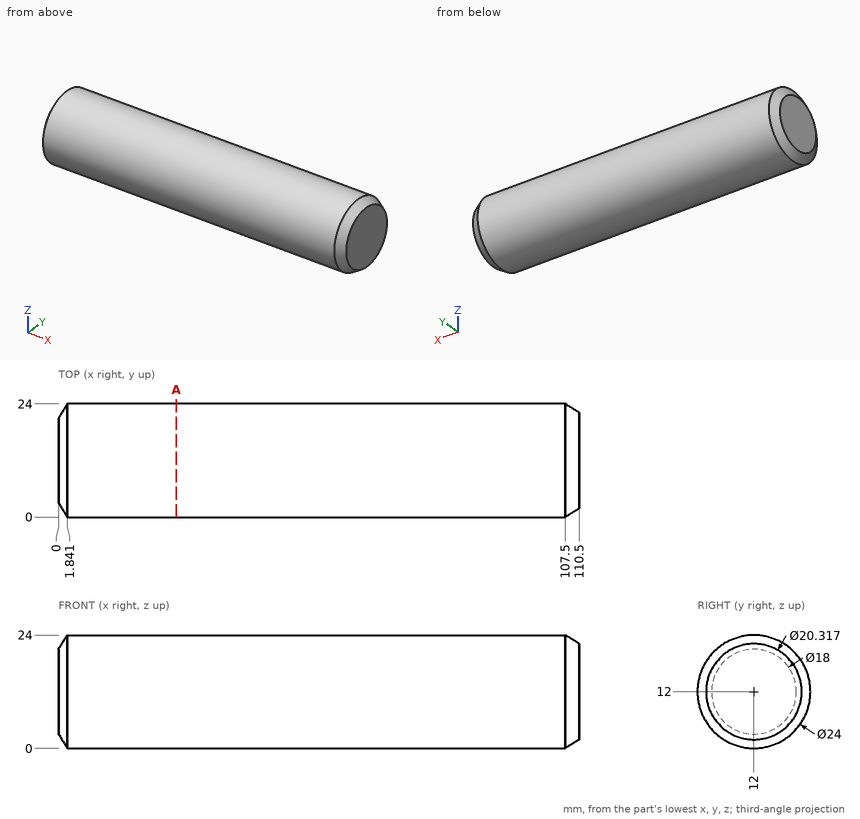
Verification items for this drawing (mm, ordinates from the low corner). Give positions to 0.01 mm unless a question says otherwise; leave off trailing zeros. Order: outer loops, then holes, each group sorted by start corner. A loop starts at its lowest first (then second) coordinate and runs counter-clockwise, first axis right, second up. Notation, with made-up numbers: M 63,54 L 98,54 A15 ccw 98,71 Z; hole C 6.25,-25 d7. An arc over 180 degrees is marked long. Use a Markdown table: item, result.
Item 1: Section check A-A (x = 25). Record the cut outline in (y, z).
Answers follow:
| item | result |
|---|---|
| outline | C 12,12 d24 |
Item 2: Material ranges on line 1 along Y through (x, z) = (102.5, 4) (1 decimal); line 2 along Y through (x, z) = (48.5, 6); line 3 along Z through (x, y) = (81.5, 12.25), recorded low to high.
Answers follow:
| item | result |
|---|---|
| line 1 | y = 3.1 to 20.9 |
| line 2 | y = 1.61 to 22.39 |
| line 3 | z = 0 to 24 |
Item 3: Depth check by flat-ended pin: P1, Ø12, axis at y = 18, z = 5.5, coming from the -X side; P2, Ø4, axis at x = 68.5, y = 9, coming from the +Z side; P3, Ø2, axis at x = 83.5, z = 5.5, coming from the -Y side (1 decimal); P4, Ø1.5, axis at y = 18.5, z = 3.5, coming from the -X side. Enter the tip coordinate at first touch or a pass-through.
Answers follow:
| item | result |
|---|---|
| P1 | stops at x = 0 |
| P2 | stops at z = 23.96 |
| P3 | stops at y = 1.3 |
| P4 | stops at x = 0.58 |
